from build123d import *

# Parameters (mm, degrees)
SKETCH1_R               = 2.2
SKETCH1_R_2             = 1.1
BOSS_EXTRUDE3_DEPTH     = 8
BOSS_EXTRUDE3_2_DEPTH   = 8
BOSS_EXTRUDE4_DEPTH     = 20
BOSS_EXTRUDE8_DEPTH     = 1
SKETCH2_W               = 24.2
SKETCH2_H               = 9.5
CUT_EXTRUDE2_DEPTH      = 9
SKETCH1_11_R            = 2.2
SKETCH1_11_R_2          = 1.1
BOSS_EXTRUDE9_DEPTH     = 8
CUT_EXTRUDE3_DEPTH      = 58
CUT_EXTRUDE3_DEPTH_BACK = 52
SKETCH3_R               = 1.5
CUT_EXTRUDE4_DEPTH      = 52
CUT_EXTRUDE4_DEPTH_BACK = 10
SKETCH4_R               = 1.5


with BuildPart() as part:
    # Sketch1 → Boss-Extrude3 (new body)
    with BuildSketch(Plane(origin=(0, 0, 0), x_dir=(1, 0, 0), z_dir=(0, 1, 0))):
        with Locations(Location((-20, 11.9, 0), (0, 0, 270))):
            Circle(SKETCH1_R)
        with Locations(Location((-20, 11.9, 0), (0, 0, 270))):
            Circle(SKETCH1_R_2, mode=Mode.SUBTRACT)
    extrude(amount=BOSS_EXTRUDE3_DEPTH)



with BuildPart() as body_2:
    # Sketch1 → Boss-Extrude3 2 (new body)
    with BuildSketch(Plane(origin=(0, 0, 0), x_dir=(1, 0, 0), z_dir=(0, 1, 0))):
        with Locations(Location((20, 11.9, 0), (0, 0, 270))):
            Circle(SKETCH1_R)
        with Locations(Location((20, 11.9, 0), (0, 0, 270))):
            Circle(SKETCH1_R_2, mode=Mode.SUBTRACT)
    extrude(amount=BOSS_EXTRUDE3_2_DEPTH)


with BuildPart() as body_3:
    # Sketch1<6> → Boss-Extrude4 (new body)
    with BuildSketch(Plane(origin=(0, 0, 0), x_dir=(1, 0, 0), z_dir=(0, 1, 0))):
        with BuildLine():
            Line((12.480384609, 36.42101042), (-12.480384609, 36.42101042))
            ThreePointArc((-12.480384609, 36.42101042), (0, -38.5), (12.480384609, 36.42101042))
        make_face()
        with BuildLine():
            ThreePointArc((-12.480384609, 34.660769231), (0, -36.839230769), (12.480384609, 34.660769231))
            Line((12.480384609, 34.660769231), (-12.480384609, 34.660769231))
        make_face(mode=Mode.SUBTRACT)
    extrude(amount=BOSS_EXTRUDE4_DEPTH)


with BuildPart() as part_1:
    add(part.part)

    add(body_2.part)  # Boss-Extrude8 merges body 2

    add(body_3.part)  # Boss-Extrude8 merges body 3
    # Sketch1<10> → Boss-Extrude8 (add)
    with BuildSketch(Plane(origin=(0, 0, 0), x_dir=(1, 0, 0), z_dir=(0, 1, 0))):
        with BuildLine():
            Line((12.480384609, 36.42101042), (-12.480384609, 36.42101042))
            ThreePointArc((-12.480384609, 36.42101042), (0, -38.5), (12.480384609, 36.42101042))
        make_face()
    extrude(amount=-BOSS_EXTRUDE8_DEPTH)

    # Sketch2 → Cut-Extrude2 (cut)
    with BuildSketch(Plane.XY.offset(-34.660769231)):
        with Locations((0, 12.25)):
            Rectangle(SKETCH2_W, SKETCH2_H)
    extrude(amount=-CUT_EXTRUDE2_DEPTH, mode=Mode.SUBTRACT)

    # Sketch1<11> → Boss-Extrude9 (add)
    with BuildSketch(Plane(origin=(0, 0, 0), x_dir=(1, 0, 0), z_dir=(0, 1, 0))):
        with Locations(Location((7.6, -26.129462263, 0), (0, 0, 270))):
            Circle(SKETCH1_11_R)
        with Locations(Location((7.6, -26.129462263, 0), (0, 0, 270))):
            Circle(SKETCH1_11_R_2, mode=Mode.SUBTRACT)
    extrude(amount=BOSS_EXTRUDE9_DEPTH)

    # Sketch3 → Cut-Extrude3 (cut, two sides: drawn at the far end of the back side and taken through both)
    with BuildSketch(Plane(origin=(0, 0, 0), x_dir=(0, 0, -1), z_dir=(1, 0, 0)).offset(-CUT_EXTRUDE3_DEPTH_BACK)):
        with Locations(Location((0, 14, 0), (0, 0, 180))):
            Circle(SKETCH3_R)
    extrude(amount=CUT_EXTRUDE3_DEPTH + CUT_EXTRUDE3_DEPTH_BACK, mode=Mode.SUBTRACT)

    # Sketch4 → Cut-Extrude4 (cut, two sides: drawn at the far end of the back side and taken through both)
    with BuildSketch(Plane.XY.offset(-CUT_EXTRUDE4_DEPTH_BACK)):
        with Locations((0, 14)):
            Circle(SKETCH4_R)
    extrude(amount=CUT_EXTRUDE4_DEPTH + CUT_EXTRUDE4_DEPTH_BACK, mode=Mode.SUBTRACT)


solid = part_1.part
Read the model definition and answer for the solid it produces. Units are mm, in the model's axes. A direction names the side the tool comes from. Give positions to 0.01 mm unless a question says otherwise; leave off trailing zeros. Write each loop counter-clockwise with the first axis right and the second up, starting at its lowest first coordinate (ties: lowest second). Pieces come first, ordered by that corner, then holes. Notation, with made-up numbers: (60.5, 33.25) - (87.5, 33.25) arc R23 cw to (87.5, 58.25) - close; hole circle Ø9 at (-20.5, -24). An arc over 180 degrees is marked (long way). Use CSV: the item, a comma, the result in double quotes. Start each with the question number.
(1) For faces 1 (the cylindrical face through (-0.325, 12.536, 37.642)), 2 (the cylindrical face through (-1.44, 9.86, 36.81)), 3 (the flat face through (12.1, 12, -36)), determine the directions among +Z, -Z, +X, -X, +Y, -Y from which every point of the face is accessible in a straight line to the end or side of a thin tool.
(2) Find section D-D (y = 10.75). Give the vertices of the cut face in (x, z), plus the area to 3 significant figures.
(3) Determine the mould class of faces 4 (the flat face through (3, 20, -35)), 5 (the flat face through (-1, 0, 1)) for opening direction X: +X half, -X half, draft (parallel to the pull), parting line (faces both ways), or undercut.
(4) Find section B-B (x = 0). Give the vertices of the cut face in (y, z), plus the area to 3 significant figures.
(5) Consider line 1 along Y through (x, z) = (-37, 0); line 2 along Y through (x, z) = (18, 22.5); line 3 along X through (y, z) = (5.5, 23.5). Determine where each line is inside the solid, lowest interval first.
(6) Find section C-C (z = 0). Give the vertices of the cut face in (x, y).
(7) Given P1, Ø12, axis at y = 7.5, z = -10, coming from the -X side; P2, Ø3.5, axis at x = 20, z = -11.5, coming from the +Y side; P3, Ø1.4, axis at y = 14.5, z = -36, coming from the +X side; P4, Ø2.5, axis at y = 14, z = 0, coming from the -X side, each flat-ended and moving along its own axis, determine where each tip first touches the part or whether it passes through.
(8) Find section A-A (y = 3.25). Give the vertices of the cut face in (x, z).
Findings below:
1,face 1,"+Z, -Z"
1,face 2,"+Y"
1,face 3,"-Z"
2,outline,"(-12.48, -36.42) - (-12.1, -36.42) - (-12.1, -34.66) - (-12.48, -34.66) arc R36.84 cw (long way) to (12.48, -34.66) - (12.1, -34.66) - (12.1, -36.42) - (12.48, -36.42) arc R38.5 ccw (long way) to start"
2,area,"352 mm2"
3,face 4,"draft"
3,face 5,"undercut"
4,outline,"(-1, -36.42) - (7.5, -36.42) - (7.5, -34.66) - (0, -34.66) - (0, 36.84) - (12.5, 36.84) - (12.5, 38.5) - (-1, 38.5) - close; (15.5, 36.84) - (20, 36.84) - (20, 38.5) - (15.5, 38.5) - close; (17, -36.42) - (20, -36.42) - (20, -34.66) - (17, -34.66) - close"
4,area,"122 mm2"
5,line 1,"-1 to 12.5, 15.5 to 20"
5,line 2,"-1 to 0"
5,line 3,"-30.5 to -28.37, 28.37 to 30.5"
6,outline,"(-38.5, -1) - (38.5, -1) - (38.5, 12.5) - (36.84, 12.5) - (36.84, 0) - (-36.84, 0) - (-36.84, 12.5) - (-38.5, 12.5) - close; (-38.5, 15.5) - (-36.84, 15.5) - (-36.84, 20) - (-38.5, 20) - close; (36.84, 15.5) - (38.5, 15.5) - (38.5, 20) - (36.84, 20) - close"
7,P1,"x = -38.29"
7,P2,"y = 8"
7,P3,"x = 15.37"
7,P4,"through"
8,outline,"circle Ø4.4 at (-20, -11.9); (-12.48, -36.42) - (12.48, -36.42) arc R38.5 ccw (long way) to start; circle Ø4.4 at (7.6, 26.13); circle Ø4.4 at (20, -11.9); hole circle Ø2.2 at (-20, -11.9); hole (-12.48, -34.66) - (12.48, -34.66) arc R36.84 ccw (long way) to start; hole circle Ø2.2 at (7.6, 26.13); hole circle Ø2.2 at (20, -11.9)"
